from build123d import *

# Parameters (mm, degrees)
F1_DEPTH  = 12.7
F2_DEPTH  = 2.54
F3_R      = 6
F4_R      = 7.2644
F5_R      = 2.54
F6_DEPTH  = 25.4
F6_TAPER  = -45
F0_W      = 9.144
F0_H      = 1.27
F7_DEPTH  = 6.35
F0_W_2    = 25.908
F8_DEPTH  = 2.54
F9_R      = 2.54
F10_DEPTH = 0.762


with BuildPart() as f1:
    # F0 (on Front) → F1 (new body)
    with BuildSketch(Plane.XZ):
        Polygon((-47.625, 13.97), (-69.723, 13.97), (-69.723, -13.97), (69.723, -13.97), (69.723, 13.97), (47.625, 13.97), (47.625, 12.7), (68.453, 12.7), (68.453, -12.7), (2.5605612715, -12.7), (-2.5605612715, -12.7), (-68.453, -12.7), (-68.453, 12.7), (-47.625, 12.7), align=None)
    extrude(amount=F1_DEPTH)

    # F0 (on Front) → F2 (join)
    with BuildSketch(Plane.XZ):
        Polygon((-21.717, 12.7), (-47.625, 12.7), (-68.453, 12.7), (-68.453, -12.7), (-2.5605612715, -12.7), (-4.782773325, 12.7), (-12.573, 12.7), align=None)
        Polygon((68.453, 12.7), (47.625, 12.7), (21.717, 12.7), (12.573, 12.7), (4.782773325, 12.7), (2.5605612715, -12.7), (68.453, -12.7), align=None)
    extrude(amount=F2_DEPTH)

    # F3
    f3_edges = [f1.edges().sort_by_distance(p)[0] for p in [
        (-68.453, -7.62, 12.7),
        (-68.453, -7.62, -12.7),
        (68.453, -7.62, 12.7),
        (68.453, -7.62, -12.7),
    ]]
    fillet(f3_edges, radius=F3_R)

    # F4
    f4_edges = [f1.edges().sort_by_distance(p)[0] for p in [
        (-69.723, -6.35, 13.97),
        (-69.723, -6.35, -13.97),
        (69.723, -6.35, -13.97),
        (69.723, -6.35, 13.97),
    ]]
    fillet(f4_edges, radius=F4_R)

    # F5 (on face) → F6 (cut)
    with BuildSketch(Plane.XZ.offset(2.54)):
        with Locations((-38.1, 0)):
            Circle(F5_R)
        with Locations((38.1, 0)):
            Circle(F5_R)
    extrude(amount=-F6_DEPTH, taper=F6_TAPER, mode=Mode.SUBTRACT)

    # F0 (on Front) → F7 (join)
    with BuildSketch(Plane.XZ):
        with Locations((17.145, 13.335)):
            Rectangle(F0_W, F0_H)
        with Locations((-17.145, 13.335)):
            Rectangle(F0_W, F0_H)
    extrude(amount=F7_DEPTH)

    # F0 (on Front) → F8 (join)
    with BuildSketch(Plane.XZ):
        with Locations((34.671, 13.335)):
            Rectangle(F0_W_2, F0_H)
        Polygon((12.573, 13.97), (4.8938839277, 13.97), (4.782773325, 12.7), (12.573, 12.7), align=None)
        with Locations((-34.671, 13.335)):
            Rectangle(F0_W_2, F0_H)
        Polygon((-4.8938839277, 13.97), (-12.573, 13.97), (-12.573, 12.7), (-4.782773325, 12.7), align=None)
    extrude(amount=F8_DEPTH)

    # F9
    f9_edges = [f1.edges().sort_by_distance(p)[0] for p in [
        (47.625, -12.7, 13.335),
        (21.717, -6.35, 13.335),
        (12.573, -6.35, 13.335),
        (-12.573, -6.35, 13.335),
        (-21.717, -6.35, 13.335),
        (-47.625, -12.7, 13.335),
    ]]
    fillet(f9_edges, radius=F9_R)

    # F0 (on Front) → F10 (join)
    with BuildSketch(Plane.XZ):
        Polygon((4.782773325, 12.7), (-4.782773325, 12.7), (-2.5605612715, -12.7), (2.5605612715, -12.7), align=None)
        Polygon((4.8938839277, 13.97), (-4.8938839277, 13.97), (-4.782773325, 12.7), (4.782773325, 12.7), align=None)
    extrude(amount=F10_DEPTH)


solid = f1.part
The listing builds one solid part. Answer for the finished solid, in the listing's coordinates (mm). A direction names the side the tool comes from. Give positions to 0.01 mm unless a question says otherwise; leave off trailing zeros. Order: outer loops, then holes, each group sorted by start corner. A loop starts at its lowest first (then second) coordinate and runs counter-clockwise, first axis right, second up. Notation, with made-up numbers: (24.5, -35) - (69.5, -35) arc R22 ccw to (69.5, -8) - close; hole circle Ø5 at (29.5, 52). An arc over 180 degrees is marked (long way). One line per item, written item: value. Start each with the question number.
1) A cutting plane is placed at B-B on y = -7.5. Give the vertices of the cut face in (x, z) (3 decimals).
2) A cutting plane is placed at D-D on x = -8.5. Give the vertices of the cut face in (y, z).
3) A tool of negligible diameter and unlimited length cuts with its end or side. For faces 1 (the face through (-13.34, -5.63, 13.34)), 2 (the face through (67.651, -6.439, -11.786)), 3 (the face through (-66.65, -7.69, -10.99)), from which of +Z, -Z, +X, -X, +Y, -Y can it reach the whole face along a straight path? Write none if from no direction.
4) A cutting plane is placed at A-A on x = 38.1. Give the vertices of the cut face in (y, z).
5) A cutting plane is placed at C-C on z = 9.25. Give the vertices of the cut face in (x, y), then the cut area to 3 significant figures.
6) Given pin 1 Ø0.6 at (x, z) = (-17.5, 13.5) entering from -Y; pin 2 Ø1.4 at (y, z) = (-7, 13.5) entering from -X; pin 3 Ø0.6 at (y, z) = (-3, 13.5) entering from -X, each flat-ended and moving along its own axis, determine where each tip first touches the part or whether it passes through.
7) The mould has two halves that part along Z. Classify faces 4 (the face through (-1, -6, -13.97)), 5 (the face through (67.539, -6.439, 11.898)), 6 (the face through (55, -8, 12.7)): released by +Z, released by -Z, zero draft, split by the parting line, or undercut.
8) Find the intervals of material crossed by L1, parallel to Z at x = 56, y = -5.25; L2, parallel to X at y = -9.75, z = 5; L3, parallel to Y at x = -43, z = 2, in increasing order.
Answer sheet:
1. outline: (-69.723, -6.706) arc R7.264 ccw to (-62.459, -13.97) - (62.459, -13.97) arc R7.264 ccw to (69.723, -6.706) - (69.723, 6.706) arc R7.264 ccw to (62.459, 13.97) - (47.625, 13.97) - (47.625, 12.7) - (62.453, 12.7) arc R6 cw to (68.453, 6.7) - (68.453, -6.7) arc R6 cw to (62.453, -12.7) - (-62.453, -12.7) arc R6 cw to (-68.453, -6.7) - (-68.453, 6.7) arc R6 cw to (-62.453, 12.7) - (-47.625, 12.7) - (-47.625, 13.97) - (-62.459, 13.97) arc R7.264 ccw to (-69.723, 6.706) - close
2. outline: (-12.7, -13.97) - (0, -13.97) - (0, 13.97) - (-2.54, 13.97) - (-2.54, -12.7) - (-12.7, -12.7) - close
3. face 1: +Z, -Y
3. face 2: -Z, +X, +Y, -Y
3. face 3: -Y
4. outline: (-12.7, -13.97) - (0, -13.97) - (0, -5.08) - (-2.54, -2.54) - (-2.54, -12.7) - (-12.7, -12.7) - close; (-2.54, 2.54) - (0, 5.08) - (0, 13.97) - (-2.54, 13.97) - close
5. outline: (-69.26, -12.7) - (-67.88, -12.7) - (-67.88, -2.54) - (-4.48, -2.54) - (-4.48, -0.76) - (4.48, -0.76) - (4.48, -2.54) - (67.88, -2.54) - (67.88, -12.7) - (69.26, -12.7) - (69.26, 0) - (-69.26, 0) - close
5. area: 364 mm2
6. pin 1: stops at y = -6.35
6. pin 2: stops at x = -66.41
6. pin 3: stops at x = -65.71
7. face 4: released by -Z
7. face 5: released by +Z
7. face 6: undercut
8. L1: z = -13.97 to -12.7, 12.7 to 13.97
8. L2: x = -69.72 to -68.45, 68.45 to 69.72
8. L3: y = -2.54 to 0
